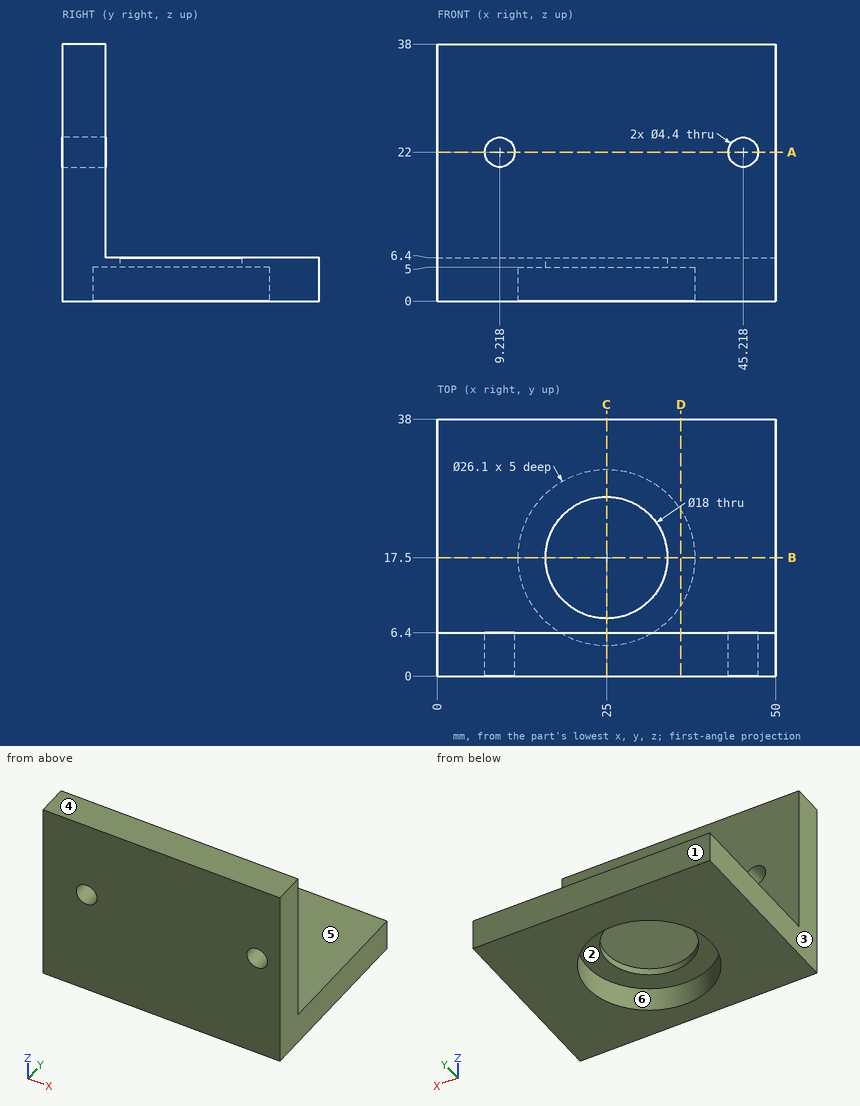
Can you work these out from the drawing? Everything is in mm from the part's minimum corner. A direction names the side the tool comes from. Give positions to 0.01 mm unless a question says otherwise; leave off trailing zeros. Order: outer loops, then holes, each group sorted by start corner. A loop starts at its lowest first (then second) coordinate and runs counter-clockwise, first axis right, second up.
1. Suppose I cut it at C-C (x = 25). List the corners of the cut face in (y, z) for me.
2. Will these pins go through, and if not, where does the flat tip stop? P1, Ø12, axis at y = 17.5, z = 12.5, coming from the +X side; P2, Ø10, axis at x = 27.5, z = 18.5, coming from the +Y side; P3, Ø16, axis at x = 29.5, y = 24, coming from the +Z side; P4, Ø13, axis at x = 22.5, y = 12.5, coming from the -Z side.
3. Suppose I cut it at D-D (x = 36). List the corners of the cut face in (y, z) for me.
4. We'd pull the mould along X, two halves only. Please class the marked faces 1, 2 and 3: pulls with the +X half, pulls with the -X half, needs draft (parallel to the pull), parting line crosses it, or undercut.
5. For the marked faces 4, 5 and 6, which set-ups out of +Z, -Z, +X, -X, +Y, -Y let a thin tool reach every point of the face, with its end or its side?
6. I need wall thicknesses on L1, parallel to X at y = 2, z = 22; L2, parallel to Y at x = 25, z = 2; L3, parallel to X at y = 2, z = 21.5 (1 decimal). Which ranges of each line are inside material? Lowest first, please.
7. Suppose I cut it at B-B (y = 17.5). List the corners of the cut face in (x, z) for me, plus the area to 3 significant figures.
8. Suppose I cut it at A-A (z = 22). List the corners of the cut face in (x, y) for me.
Solved:
1. outline: (0, 0) - (4.45, 0) - (4.45, 5) - (8.5, 5) - (8.5, 6.4) - (6.4, 6.4) - (6.4, 38) - (0, 38) - close; (26.5, 5) - (30.55, 5) - (30.55, 0) - (38, 0) - (38, 6.4) - (26.5, 6.4) - close
2. P1: passes through
2. P2: stops at y = 6.4
2. P3: stops at z = 6.4
2. P4: stops at z = 5
3. outline: (0, 0) - (10.48, 0) - (10.48, 5) - (24.52, 5) - (24.52, 0) - (38, 0) - (38, 6.4) - (6.4, 6.4) - (6.4, 38) - (0, 38) - close
4. face 1: needs draft
4. face 2: undercut
4. face 3: pulls with the -X half
5. face 4: +Z, +X, -X, +Y, -Y
5. face 5: +Z, +X, -X, +Y
5. face 6: -Z
6. L1: x = 0 to 7.02, 11.42 to 43.02, 47.42 to 50
6. L2: y = 0 to 4.45, 30.55 to 38
6. L3: x = 0 to 7.1, 11.4 to 43.1, 47.4 to 50
7. outline: (0, 0) - (11.95, 0) - (11.95, 5) - (16, 5) - (16, 6.4) - (0, 6.4) - close; (34, 5) - (38.05, 5) - (38.05, 0) - (50, 0) - (50, 6.4) - (34, 6.4) - close
7. area: 164 mm2
8. outline: (0, 0) - (7.02, 0) - (7.02, 6.4) - (0, 6.4) - close; (11.42, 0) - (43.02, 0) - (43.02, 6.4) - (11.42, 6.4) - close; (47.42, 0) - (50, 0) - (50, 6.4) - (47.42, 6.4) - close
